Geometry: final body of the model. Coordinates: model frame, mm. A direction names the side the tool comes from. Give positions to 0.01 mm unless a question says otherwise; leave off trailing zeros. Write each loop counter-clockwise with the first axis right and the second up, starting at its lowest first coordinate (ties: lowest second). Pieces come first, ordered by that corner, then holes. Notation, with made-up numbers: (-1, 21) - (8, 21) arc R5 cw to (8, 26) - close; hole circle Ø3 at (-21.5, -22.75). An arc over 180 degrees is marked (long way). Return JSON: item names as keys, results as strings.
from build123d import *

# Parameters (mm, degrees)
SKETCH1_R           = 20
BOSS_EXTRUDE1_DEPTH = 120


with BuildPart() as part:
    # Sketch1 → Boss-Extrude1 (new body)
    with BuildSketch(Plane(origin=(0, 0, 0), x_dir=(1, 0, 0), z_dir=(0, 1, 0))):
        with BuildLine():
            Line((-10, 81.215728753), (-10, 59.160797831))
            ThreePointArc((-10, 59.160797831), (-30, 51.961524227), (-46.23475383, 38.240652953))
            Line((-46.23475383, 38.240652953), (-65.334884287, 49.268118414))
            ThreePointArc((-65.334884287, 49.268118414), (-120.810543828, 69.75), (-75.334884287, 31.947610338))
            Line((-75.334884287, 31.947610338), (-56.23475383, 20.920144878))
            ThreePointArc((-56.23475383, 20.920144878), (-60, 0), (-56.23475383, -20.920144878))
            Line((-56.23475383, -20.920144878), (-75.334884287, -31.947610338))
            ThreePointArc((-75.334884287, -31.947610338), (-120.810543828, -69.75), (-65.334884287, -49.268118414))
            Line((-65.334884287, -49.268118414), (-46.23475383, -38.240652953))
            ThreePointArc((-46.23475383, -38.240652953), (-30, -51.961524227), (-10, -59.160797831))
            Line((-10, -59.160797831), (-10, -81.215728753))
            ThreePointArc((-10, -81.215728753), (0, -139.5), (10, -81.215728753))
            Line((10, -81.215728753), (10, -59.160797831))
            ThreePointArc((10, -59.160797831), (30, -51.961524227), (46.23475383, -38.240652953))
            Line((46.23475383, -38.240652953), (65.334884287, -49.268118414))
            ThreePointArc((65.334884287, -49.268118414), (120.810543828, -69.75), (75.334884287, -31.947610338))
            Line((75.334884287, -31.947610338), (56.23475383, -20.920144878))
            ThreePointArc((56.23475383, -20.920144878), (60, 0), (56.23475383, 20.920144878))
            Line((56.23475383, 20.920144878), (75.334884287, 31.947610338))
            ThreePointArc((75.334884287, 31.947610338), (120.810543828, 69.75), (65.334884287, 49.268118414))
            Line((65.334884287, 49.268118414), (46.23475383, 38.240652953))
            ThreePointArc((46.23475383, 38.240652953), (30, 51.961524227), (10, 59.160797831))
            Line((10, 59.160797831), (10, 81.215728753))
            ThreePointArc((10, 81.215728753), (0, 139.5), (-10, 81.215728753))
        make_face()
        with Locations((0, 109.5)):
            Circle(SKETCH1_R, mode=Mode.SUBTRACT)
        with Locations((94.829781714, 54.75)):
            Circle(SKETCH1_R, mode=Mode.SUBTRACT)
        with Locations((94.829781714, -54.75)):
            Circle(SKETCH1_R, mode=Mode.SUBTRACT)
        with Locations((0, -109.5)):
            Circle(SKETCH1_R, mode=Mode.SUBTRACT)
        with Locations((-94.829781714, -54.75)):
            Circle(SKETCH1_R, mode=Mode.SUBTRACT)
        with Locations((-94.829781714, 54.75)):
            Circle(SKETCH1_R, mode=Mode.SUBTRACT)
        with BuildLine():
            Line((-35, 11.5), (-35, -11.5))
            Line((-35, -11.5), (-25.529394822, -11.5))
            ThreePointArc((-25.529394822, -11.5), (0, -28), (25.529394822, -11.5))
            Line((25.529394822, -11.5), (35, -11.5))
            Line((35, -11.5), (35, 11.5))
            Line((35, 11.5), (25.529394822, 11.5))
            ThreePointArc((25.529394822, 11.5), (0, 28), (-25.529394822, 11.5))
            Line((-25.529394822, 11.5), (-35, 11.5))
        make_face(mode=Mode.SUBTRACT)
    extrude(amount=BOSS_EXTRUDE1_DEPTH)


solid = part.part
Q1. Section query D-D, the plane z = -1. Return the cut outline in (x, y).
Answer key:
{"outline": "(-59.99, 0) - (-35, 0) - (-35, 120) - (-59.99, 120) - close; (35, 0) - (59.99, 0) - (59.99, 120) - (35, 120) - close"}
Q2. Mould query, pull axis Z, two halves, no side actions, for faces 1 (the flat face through (-30, 59, -11.5)), 2 (the flat face through (9, 0, 30)), 3 (the cylindrical face through (-121.38, 59.16, 68.72)). Classes: pulls with the +Z half, pulls with the -Z half, needs draft (parallel to the pull), parting line crosses it, or undercut.
Answer key:
{"face 1": "undercut", "face 2": "needs draft", "face 3": "undercut"}
Q3. Section query B-B, the plane x = -4.5. Return the cut outline in (y, z), plus the area to 3 significant figures.
Answer key:
{"outline": "(0, -139.16) - (120, -139.16) - (120, -128.99) - (0, -128.99) - close; (0, -90.01) - (120, -90.01) - (120, -27.64) - (0, -27.64) - close; (0, 27.64) - (120, 27.64) - (120, 90.01) - (0, 90.01) - close; (0, 128.99) - (120, 128.99) - (120, 139.16) - (0, 139.16) - close", "area": "17,400 mm^2"}
Q4. Set-up query: faces 4 (the flat face through (-10, 59, 70)), 5 (the cylindrical face through (60, 59, 0)). Return all of +Z, -Z, +X, -X, +Y, -Y with unobstructed straight access to the full face (end or side cutting, diameter ignored); none if empty.
Answer key:
{"face 4": "+Y, -Y", "face 5": "+X, +Y, -Y"}
Q5. Pin query (flat end, axial travel): P1, Ø11, axis at y = 68.5, z = -67, coming from the -X side; P2, Ø6, axis at x = -23, y = 40.5, coming from the +Z side; P3, Ø7.5, axis at x = -30, y = 72, coming from the -Z side. Return the tip coordinate at first contact, or that it passes through.
Answer key:
{"P1": "stops at x = -124.06", "P2": "stops at z = 131.86", "P3": "stops at z = -124.02"}
Q6. Material intervals for probe 1 along Z at (x, y) = (-94, 94); probe 2 along X at (y, z) = (69, 109.5); probe 3 along Z at (x, y) = (84, 6), sorted ascending. Write a range as [from, to].
Answer key:
{"probe 1": "z = [-84.74, -74.73], [-34.77, -24.76], [24.76, 34.77], [74.73, 84.74]", "probe 2": "x = [-30, -20], [20, 30]", "probe 3": "z = [-82.73, -71.56], [-37.94, -26.77], [26.77, 37.94], [71.56, 82.73]"}
Q7. Section query C-C, the plane z = -54.75. Return the cut outline in (x, y).
Answer key:
{"outline": "(-124.83, 0) - (-114.83, 0) - (-114.83, 120) - (-124.83, 120) - close; (-74.83, 0) - (-64.83, 0) - (-64.83, 120) - (-74.83, 120) - close; (-24.54, 0) - (24.54, 0) - (24.54, 120) - (-24.54, 120) - close; (64.83, 0) - (74.83, 0) - (74.83, 120) - (64.83, 120) - close; (114.83, 0) - (124.83, 0) - (124.83, 120) - (114.83, 120) - close"}
Q8. Section query A-A, the plane z = -109.5. Return the cut outline in (x, y), plus the area to 3 significant figures.
Answer key:
{"outline": "(-30, 0) - (-20, 0) - (-20, 120) - (-30, 120) - close; (20, 0) - (30, 0) - (30, 120) - (20, 120) - close", "area": "2,400 mm^2"}
